Answer from the drawing. Dimensions are ordinates in mm from the lowest x, y and z of the part. A direction names the side the tool comes from. Coordinates: 2 decimals unless noted, no trailing zeros. Loops run counter-clockwise (first coordinate to the right, second up) from the corner with the lowest first, then second, coordinate; pieces in that order, holes last.
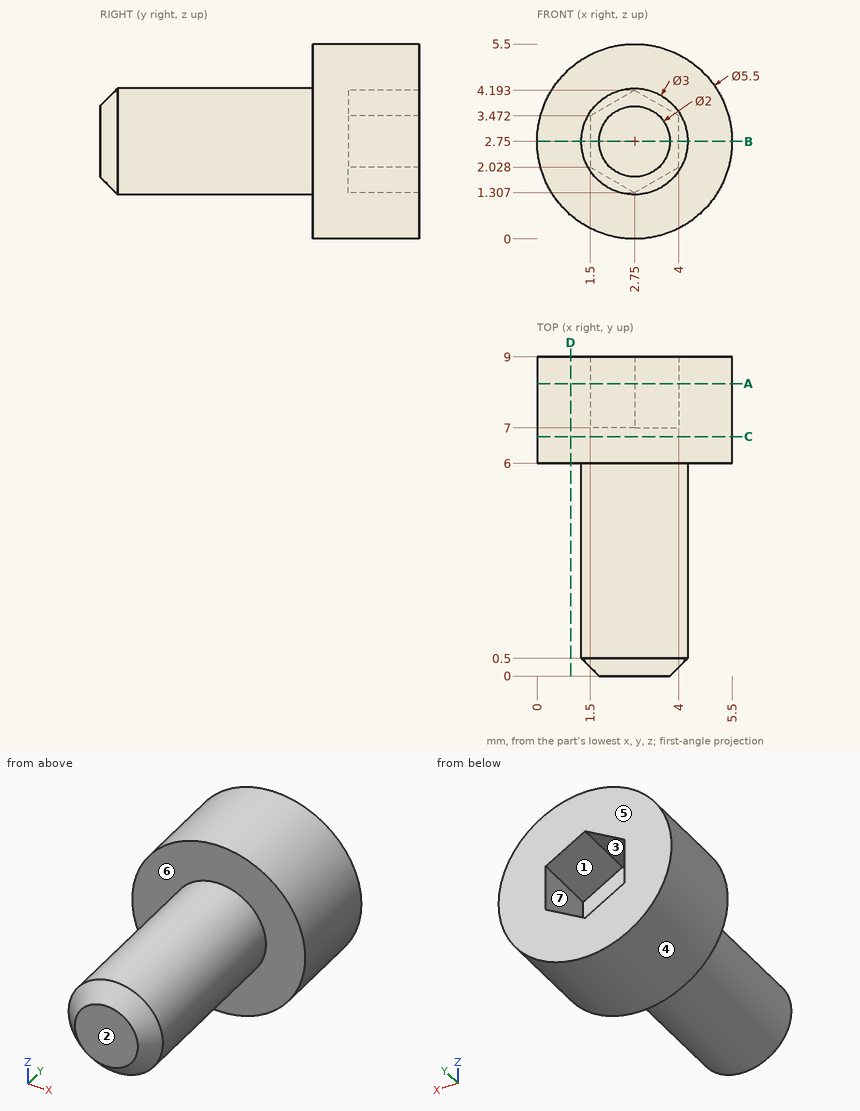
Item 1: A cutting plane is placed at C-C on y = 6.75. Determine the outline of the cut face in (x, z).
Numbers:
outline: circle Ø5.5 at (2.75, 2.75)
Item 2: A cutting plane is placed at A-A on y = 8.25. Determine the outline of the cut face in (x, z).
Numbers:
outline: circle Ø5.5 at (2.75, 2.75); hole (1.5, 2.03) - (2.75, 1.31) - (4, 2.03) - (4, 3.47) - (2.75, 4.19) - (1.5, 3.47) - close
Item 3: Determine the mould class of the marked faces 1, 2, 3 and 4 for opening direction Z: released by +Z, released by -Z, zero draft, split by the parting line, or undercut.
Numbers:
face 1: undercut
face 2: zero draft
face 3: undercut
face 4: split by the parting line
Item 4: A cutting plane is placed at D-D on x = 0.95. Determine the outline of the cut face in (y, z), then the cut area to 3 significant figures.
Numbers:
outline: (6, 0.67) - (9, 0.67) - (9, 4.83) - (6, 4.83) - close
area: 12.5 mm2
Item 5: A cutting plane is placed at B-B on z = 2.75. Determine the outline of the cut face in (x, y).
Numbers:
outline: (0, 6) - (1.25, 6) - (1.25, 0.5) - (1.75, 0) - (3.75, 0) - (4.25, 0.5) - (4.25, 6) - (5.5, 6) - (5.5, 9) - (4, 9) - (4, 7) - (1.5, 7) - (1.5, 9) - (0, 9) - close
Item 6: Find the intervals of material crossed by line 1 along X through (y, z) = (7.75, 2.85); line 2 along Y through (x, z) = (1.35, 3.65); line 3 along X through (y, z) = (2.5, 3.15) (1 decimal), in increasing order.
Numbers:
line 1: x = 0 to 1.5, 4 to 5.5
line 2: y = 6 to 9
line 3: x = 1.3 to 4.2
Item 7: Given pin 1 (2 mm diameter, centred on x = 5, y = 2, fed in from +Z); pin 2 (1 mm diameter, centred on x = 3, y = 1.5, fed in from -Z), each flat-ended and moving along its own axis, determine where each tip first touches the part or whether it passes through.
Numbers:
pin 1: stops at z = 3.58
pin 2: stops at z = 1.25
Item 8: Which of the six approach directions +Z, -Z, +X, -X, +Y, -Y give full straight-line access (tool end or side, diameter ignored) to the marked faces 5, 6 and 7?
Numbers:
face 5: +Z, -Z, +X, -X, +Y
face 6: -Y
face 7: +Y
